Geometry check sheet. Reference: the model listing, model coordinates, mm. A direction names the side the tool comes from. Give positions to 0.01 mm unless a question says otherwise; leave off trailing zeros. Loops run counter-clockwise (first coordinate to the right, second up) from the corner with the lowest first, then second, coordinate; pieces in that order, holes last. Notation, with made-up numbers: (89, 19.5) -> (109, 19.5) arc R14 cw to (109, 35.5) -> close; hole circle Ø9 at (82.5, 51.5). An arc over 180 degrees is marked (long way). Write item = value, one per line.
```python
from build123d import *

# Parameters (mm, degrees)
SKETCH_1_R          = 6
EXTRUDE_1_DEPTH     = 4
SKETCH_2_R          = 4
EXTRUDE_2_DEPTH     = 21
SKETCH_3_R          = 3
EXTRUDE_3_DEPTH     = 6
SKETCH_4_R          = 7.5
SKETCH_4_W          = 10
SKETCH_4_H          = 10
CUT_EXTRUDE_1_DEPTH = 6


with BuildPart() as part:
    # 草图1 → 凸台-拉伸1 (new body)
    with BuildSketch(Plane.XY):
        Circle(SKETCH_1_R)
    extrude(amount=EXTRUDE_1_DEPTH)

    # 草图2 → 凸台-拉伸2 (add)
    with BuildSketch(Plane.XY.offset(4)):
        Circle(SKETCH_2_R)
    extrude(amount=EXTRUDE_2_DEPTH)

    # 草图3 → 凸台-拉伸3 (add)
    with BuildSketch(Plane.XY.offset(25)):
        Circle(SKETCH_3_R)
    extrude(amount=EXTRUDE_3_DEPTH)

    # 草图4 → 切除-拉伸1 (cut)
    with BuildSketch(Plane(origin=(0, 0, 0), x_dir=(-1, 0, 0), z_dir=(0, 0, -1))):
        Circle(SKETCH_4_R)
        Rectangle(SKETCH_4_W, SKETCH_4_H, mode=Mode.SUBTRACT)
    extrude(amount=-CUT_EXTRUDE_1_DEPTH, mode=Mode.SUBTRACT)


solid = part.part
```
Item 1: Tool access check on faces 1 (the cylindrical face through (4.254, 4.231, 1.972)), 2 (the flat face through (1, 3, 25)). Record the directions out of +Z, -Z, +X, -X, +Y, -Y that give a thin tool (end or side, any length) a straight path to the whole face; none if there is none.
Answer:
face_1 = +Z, -Z, +X, +Y
face_2 = +Z
Item 2: Section check A-A, the plane y = 0. Record the cut outline in (x, z).
Answer:
outline = (-5, 0) -> (5, 0) -> (5, 4) -> (4, 4) -> (4, 25) -> (3, 25) -> (3, 31) -> (-3, 31) -> (-3, 25) -> (-4, 25) -> (-4, 4) -> (-5, 4) -> close
Item 3: Section check D-D, the plane z = 25.5. Record the cut outline in (x, y), plus the area to 3 significant figures.
Answer:
outline = circle Ø6 at (0, 0)
area = 28.3 mm^2
Item 4: Thickness scan on L1, parallel to Z at x = -4, y = 3.25; L2, parallel to Z at x = -2, y = 2.5; L3, parallel to Y at x = -0.75, z = 19. Record the ranges inside material, lowest first. Write a range as [from, to].
Answer:
L1 = [0, 4]
L2 = [0, 25]
L3 = [-3.93, 3.93]
Item 5: Gauge pin test, flat ends, axial feed: pin 1 (5 mm diameter, centred on x = -3, z = 25.5, fed in from -Y); pin 2 (2 mm diameter, centred on y = 3.5, z = 23.5, fed in from -X); pin 3 (1.5 mm diameter, centred on y = -1, z = 22.5, fed in from -X). Record the tip position at first contact, or that the pin passes through.
Answer:
pin_1 = -3.96
pin_2 = -3.12
pin_3 = -3.99
Item 6: Section check C-C, the plane z = 6. Record the cut outline in (x, y).
Answer:
outline = circle Ø8 at (0, 0)
